```python
from build123d import *

# Parameters (mm, degrees)
SKETCH_1_W          = 45
SKETCH_1_H          = 30
EXTRUDE_1_DEPTH     = 40
SKETCH_2_W          = 10
SKETCH_2_H          = 3
SKETCH_2_H_2        = 2
CUT_EXTRUDE_1_DEPTH = 49.28301979
CUT_EXTRUDE_2_DEPTH = 5
CUT_EXTRUDE_3_DEPTH = 12
CUT_EXTRUDE_4_DEPTH = 63.048368391
SKETCH_6_W          = 5
SKETCH_6_H          = 10
CUT_EXTRUDE_5_DEPTH = 14.19009
EXTRUDE_2_DEPTH     = 10
SKETCH_8_W          = 12
SKETCH_8_H          = 6
CUT_EXTRUDE_6_DEPTH = 10
SKETCH_9_W          = 12
SKETCH_9_H          = 18
CUT_EXTRUDE_7_DEPTH = 10
EXTRUDE_START       = -1e-06
SKETCH_10_W         = 5
SKETCH_10_H         = 10
EXTRUDE_3_DEPTH     = 4.19009
EXTRUDE_4_DEPTH     = 10


with BuildPart() as part:
    # Эскиз1 → Бобышка-Вытянуть1 (new body)
    with BuildSketch(Plane(origin=(0, 0, 0), x_dir=(0, 0, -1), z_dir=(1, 0, 0))):
        Rectangle(SKETCH_1_W, SKETCH_1_H)
    extrude(amount=EXTRUDE_1_DEPTH)

    # Эскиз2 → Вырез-Вытянуть1 (cut, through all)
    with BuildSketch(Plane(origin=(40, 0, 0), x_dir=(0, 0, -1), z_dir=(1, 0, 0))):
        with Locations((0, -11.5)):
            Rectangle(SKETCH_2_W, SKETCH_2_H)
        with Locations((0, -14)):
            Rectangle(SKETCH_2_W, SKETCH_2_H_2)
    extrude(amount=-CUT_EXTRUDE_1_DEPTH, mode=Mode.SUBTRACT)

    # Эскиз3 → Вырез-Вытянуть2 (cut)
    with BuildSketch(Plane(origin=(40, 0, 0), x_dir=(0, 0, -1), z_dir=(1, 0, 0))):
        with BuildLine():
            Line((-22.5, 15), (-22.5, -10))
            add(Edge.make_bspline(
                [(-8.309911122, 15), (-8.309911122, 6.581189356), (-12.462330184, -5.292395359), (-22.5, -10)],
                knots=[0, 0, 0, 0, 1, 1, 1, 1], degree=3))
            Line((-8.309911122, 15), (-22.5, 15))
        make_face()
    extrude(amount=-CUT_EXTRUDE_2_DEPTH, mode=Mode.SUBTRACT)

    # Эскиз4 → Вырез-Вытянуть3 (cut)
    with BuildSketch(Plane(origin=(0, 0, -22.5), x_dir=(-1, 0, 0), z_dir=(0, 0, -1))):
        Polygon((-40, 15), (-35, 15), (-40, -10), align=None)
    extrude(amount=-CUT_EXTRUDE_3_DEPTH, mode=Mode.SUBTRACT)

    # Эскиз5 → Вырез-Вытянуть4 (cut, through all)
    with BuildSketch(Plane.XY.offset(22.5)):
        Polygon((20, -10), (30, -15), (10, -15), align=None)
    extrude(amount=-CUT_EXTRUDE_4_DEPTH, mode=Mode.SUBTRACT)

    # Эскиз6 → Вырез-Вытянуть5 (cut)
    with BuildSketch(Plane.XY.offset(22.5)):
        with Locations((2.5, 10)):
            Rectangle(SKETCH_6_W, SKETCH_6_H)
    extrude(amount=-CUT_EXTRUDE_5_DEPTH, mode=Mode.SUBTRACT)

    # Эскиз7 → Бобышка-Вытянуть2 (add)
    with BuildSketch(Plane.XY.offset(22.5)):
        Polygon((35, 15), (35, 18), (25, 23), (15, 23), (5, 18), (5, 15), align=None)
    extrude(amount=-EXTRUDE_2_DEPTH)

    # Эскиз8 → Вырез-Вытянуть6 (cut)
    with BuildSketch(Plane.ZY):
        with Locations((-16.5, 12)):
            Rectangle(SKETCH_8_W, SKETCH_8_H)
    extrude(amount=-CUT_EXTRUDE_6_DEPTH, mode=Mode.SUBTRACT)

    # Эскиз9 → Вырез-Вытянуть7 (cut)
    with BuildSketch(Plane.XY.offset(22.5)):
        with Locations((6, 14)):
            Rectangle(SKETCH_9_W, SKETCH_9_H)
    extrude(amount=-CUT_EXTRUDE_7_DEPTH, mode=Mode.SUBTRACT)

    # Эскиз10 → Бобышка-Вытянуть3 (add)
    with BuildSketch(Plane.XY.offset(8.309911122).offset(EXTRUDE_START)):
        with Locations((2.5, 10)):
            Rectangle(SKETCH_10_W, SKETCH_10_H)
    extrude(amount=EXTRUDE_3_DEPTH)

    # Эскиз11 → Бобышка-Вытянуть4 (add)
    with BuildSketch(Plane.XY.offset(22.5)):
        Polygon((15, 23), (12, 21.5), (12, 23), align=None)
    extrude(amount=-EXTRUDE_4_DEPTH)


solid = part.part
```
Source: CAD feature listing. Evaluate the final solid. Frame: model axes, mm. A direction names the side the tool comes from. Coordinates: 2 decimals unless noted, no trailing zeros. Write each loop counter-clockwise with the first axis right and the second up, starting at its lowest first coordinate (ties: lowest second). Pieces come first, ordered by that corner, then holes. Notation, with made-up numbers: M 38.25,59.5 L 71.25,59.5 A14 ccw 71.25,81.5 Z; hole C 24,74.5 d3. An arc over 180 degrees is marked long. Answer as a JSON object with one key per item and string values.
1. Cut plane A-A on y = -12. Output: boundary loops of the cut face in (x, z).
Evaluation:
{"outline": "M 0,-22.5 L 16,-22.5 L 16,-5 L 0,-5 Z; M 0,5 L 16,5 L 16,22.5 L 0,22.5 Z; M 24,-22.5 L 40,-22.5 L 40,-5 L 24,-5 Z; M 24,5 L 40,5 L 40,22.5 L 24,22.5 Z"}
2. Cut plane D-D on z = -12. Output: boundary loops of the cut face in (x, y), plus the area to 3 significant figures.
Evaluation:
{"outline": "M 0,-15 L 10,-15 L 20,-10 L 30,-15 L 40,-15 L 40,-10 L 35,15 L 10,15 L 10,9 L 0,9 Z", "area": "1,030 mm^2"}
3. Contact query for flat-ended pins moving along their axis: P1, Ø3, axis at x = 35, z = -9.5, coming from the +Y side; P2, Ø1.8, axis at y = 11.5, z = -16, coming from the -X side; P3, Ø3, axis at x = 7, y = 12.5, coming from the -Z side; P4, Ø1, axis at y = 10, z = 2.5, coming from the -X side. Output: stop coordinate, or through.
Evaluation:
{"P1": "y = 15", "P2": "x = 10", "P3": "z = -10.5", "P4": "x = 0"}
4. Ray query, L1, parallel to Z at x = 13, y = -11; L2, parallel to Y at x = 9, z = 8.5; L3, parallel to X at y = -6, z = 20.5. Return the intervals inside material, ascending.
Evaluation:
{"L1": "-22.5 to -5, 5 to 22.5", "L2": "-15 to 15", "L3": "0 to 35"}
5. Cut plane B-B on x = 26.5. Output: boundary loops of the cut face in (y, z), plus the area to 3 significant figures.
Evaluation:
{"outline": "M -13.25,-22.5 L 15,-22.5 L 15,12.5 L 22.25,12.5 L 22.25,22.5 L -13.25,22.5 L -13.25,5 L -10,5 L -10,-5 L -13.25,-5 Z", "area": "1,310 mm^2"}
6. Draft query along Z for faces 5 (the flat face through (5, 9, -17)), 6 (the flat face through (20, 0, -22.5)), 7 (the flat face through (20, -10, 0)), 8 (the flat face through (8, -13, -5)). Return one class per face: released by +Z, released by -Z, zero draft, split by the parting line, or undercut.
Evaluation:
{"face 5": "zero draft", "face 6": "released by -Z", "face 7": "undercut", "face 8": "undercut"}
7. Access query for faces 1 (the flat face through (32, -12, 5)), 2 (the flat face through (24.93, -12.465, -13.627)), 3 (the flat face through (10, 12, -17)), 4 (the flat face through (35, 7, 17)). Directions: +Z, -Z, +X, -X, +Y, -Y. A direction counts if a zero-diameter tool reaches every point of the face in a straight line with its end or side. Return the directions, or none.
Evaluation:
{"face 1": "+X, -X, -Y", "face 2": "+Z, -Z, -Y", "face 3": "-Z, -X, +Y", "face 4": "+Z, +X, +Y"}
8. Cut plane C-C on z = 6. Output: boundary loops of the cut face in (x, y).
Evaluation:
{"outline": "M 0,-15 L 10,-15 L 20,-10 L 30,-15 L 40,-15 L 40,15 L 0,15 Z"}
